```python
from build123d import *

# Parameters (mm, degrees)
BOSS_EXTRUDE1_DEPTH = 304.8
SKETCH3_R           = 2.5
CUT_EXTRUDE2_DEPTH  = 254
SKETCH8_R           = 2.5
CUT_EXTRUDE4_DEPTH  = 254
SKETCH9_R           = 2.25
CUT_EXTRUDE5_DEPTH  = 25.4


with BuildPart() as part:
    # Sketch2 → Boss-Extrude1 (new, symmetric)
    with BuildSketch(Plane.XY):
        with BuildLine():
            Line((-12.7, -12.7), (12.7, -12.7))
            Line((12.7, -12.7), (12.7, 12.7))
            Line((12.7, 12.7), (11.1125, 12.7))
            ThreePointArc((11.1125, 12.7), (9.989967985, 12.235032015), (9.525, 11.1125))
            Line((9.525, 11.1125), (9.525, -6.35))
            ThreePointArc((9.525, -6.35), (8.59506403, -8.59506403), (6.35, -9.525))
            Line((6.35, -9.525), (-11.1125, -9.525))
            ThreePointArc((-11.1125, -9.525), (-12.235032015, -9.989967985), (-12.7, -11.1125))
            Line((-12.7, -11.1125), (-12.7, -12.7))
        make_face()
    extrude(amount=BOSS_EXTRUDE1_DEPTH, both=True)

    # Sketch3 → Cut-Extrude2 (cut)
    with BuildSketch(Plane(origin=(0, 0, 0), x_dir=(1, 0, 0), z_dir=(0, 1, 0))):
        with Locations(Location((-6.35, 285.75, 0), (0, 0, 270))):
            Circle(SKETCH3_R)
        with Locations(Location((0, 292.1, 0), (0, 0, 270))):
            Circle(SKETCH3_R)
        with Locations(Location((0, 266.7, 0), (0, 0, 270))):
            Circle(SKETCH3_R)
        with Locations(Location((0, 228.6, 0), (0, 0, 270))):
            Circle(SKETCH3_R)
        with Locations(Location((0, 190.5, 0), (0, 0, 270))):
            Circle(SKETCH3_R)
        with Locations(Location((0, 152.4, 0), (0, 0, 270))):
            Circle(SKETCH3_R)
        with Locations(Location((0, 114.3, 0), (0, 0, 270))):
            Circle(SKETCH3_R)
        with Locations(Location((0, 76.2, 0), (0, 0, 270))):
            Circle(SKETCH3_R)
        with Locations(Location((0, 38.1, 0), (0, 0, 270))):
            Circle(SKETCH3_R)
        with Locations(Location((0, 0, 0), (0, 0, 270))):
            Circle(SKETCH3_R)
        with Locations(Location((0, -38.1, 0), (0, 0, 270))):
            Circle(SKETCH3_R)
        with Locations(Location((0, -76.2, 0), (0, 0, 270))):
            Circle(SKETCH3_R)
        with Locations(Location((0, -114.3, 0), (0, 0, 270))):
            Circle(SKETCH3_R)
        with Locations(Location((0, -292.1, 0), (0, 0, 270))):
            Circle(SKETCH3_R)
        with Locations(Location((-6.35, -285.75, 0), (0, 0, 270))):
            Circle(SKETCH3_R)
        with Locations(Location((0, -152.4, 0), (0, 0, 270))):
            Circle(SKETCH3_R)
        with Locations(Location((0, -190.5, 0), (0, 0, 270))):
            Circle(SKETCH3_R)
        with Locations(Location((0, -228.6, 0), (0, 0, 270))):
            Circle(SKETCH3_R)
        with Locations(Location((0, -266.7, 0), (0, 0, 270))):
            Circle(SKETCH3_R)
    extrude(amount=-CUT_EXTRUDE2_DEPTH, mode=Mode.SUBTRACT)

    # Sketch8 → Cut-Extrude4 (cut)
    with BuildSketch(Plane(origin=(12.7, 0, -12.7), x_dir=(0, 0, 1), z_dir=(-1, 0, 0))):
        with Locations(Location((295.275, 6.35, 0), (0, 0, 90))):
            Circle(SKETCH8_R)
        with Locations(Location((301.625, 0, 0), (0, 0, 90))):
            Circle(SKETCH8_R)
        with Locations(Location((279.4, 0, 0), (0, 0, 90))):
            Circle(SKETCH8_R)
        with Locations(Location((241.3, 0, 0), (0, 0, 90))):
            Circle(SKETCH8_R)
        with Locations(Location((203.2, 0, 0), (0, 0, 90))):
            Circle(SKETCH8_R)
        with Locations(Location((165.1, 0, 0), (0, 0, 90))):
            Circle(SKETCH8_R)
        with Locations(Location((127, 0, 0), (0, 0, 90))):
            Circle(SKETCH8_R)
        with Locations(Location((88.9, 0, 0), (0, 0, 90))):
            Circle(SKETCH8_R)
        with Locations(Location((50.8, 0, 0), (0, 0, 90))):
            Circle(SKETCH8_R)
        with Locations(Location((12.7, 0, 0), (0, 0, 90))):
            Circle(SKETCH8_R)
        with Locations(Location((-25.4, 0, 0), (0, 0, 90))):
            Circle(SKETCH8_R)
        with Locations(Location((-63.5, 0, 0), (0, 0, 90))):
            Circle(SKETCH8_R)
        with Locations(Location((-101.6, 0, 0), (0, 0, 90))):
            Circle(SKETCH8_R)
        with Locations(Location((-276.225, 0, 0), (0, 0, 90))):
            Circle(SKETCH8_R)
        with Locations(Location((-269.875, 6.35, 0), (0, 0, 90))):
            Circle(SKETCH8_R)
        with Locations(Location((-139.7, 0, 0), (0, 0, 90))):
            Circle(SKETCH8_R)
        with Locations(Location((-177.8, 0, 0), (0, 0, 90))):
            Circle(SKETCH8_R)
        with Locations(Location((-215.9, 0, 0), (0, 0, 90))):
            Circle(SKETCH8_R)
        with Locations(Location((-254, 0, 0), (0, 0, 90))):
            Circle(SKETCH8_R)
    extrude(amount=CUT_EXTRUDE4_DEPTH, mode=Mode.SUBTRACT)

    # Sketch9 → Cut-Extrude5 (cut)
    with BuildSketch(Plane(origin=(0, -12.7, 0), x_dir=(0, 0, -1), z_dir=(0, 1, 0))):
        with Locations(Location((-16, 0, 0), (0, 0, 270))):
            Circle(SKETCH9_R)
        with Locations(Location((16, 0, 0), (0, 0, 270))):
            Circle(SKETCH9_R)
    extrude(amount=CUT_EXTRUDE5_DEPTH, mode=Mode.SUBTRACT)


solid = part.part
```
CAD build for the part. Positions are in the model's coordinates, mm. A direction names the side the tool comes from. Coordinates: 2 decimals unless noted, no trailing zeros. Use a Markdown table: item, result. Add a question column.
(1) Drill centre lines: line 1 along X through (y, z) = (-11.2, 16); line 2 along Y through (x, z) = (4, -186.5) (3 decimals); line 3 along X through (y, z) = (4, -199) (3 decimals). Where is each one in solid material? Low to high. Write a range as [from, to].
(2) Which spindle directions (+Z, -Z, +X, -X, +Y, -Y) get a long thin tool onto all of the face, cutting with end or side? Do faces 1 (the face through (-2, -9.525, 4)), 2 (the face through (0, -12.7, 4)). Say none if no direction does.
(3) Flat gauge pins, fed straight in: pin 1 (6.5 mm diameter, centred on y = 6.35, z = 282.575, fed in from +X); pin 2 (2 mm diameter, centred on x = 3.5, z = -150.5, fed in from +Y) (3 decimals); pin 3 (3 mm diameter, centred on y = 0, z = -76.2, fed in from +X); pin 4 (8 mm diameter, centred on y = 0, z = 0, fed in from -X) (3 decimals). Where does each tip first touch, or does it go through?
Solved:
| question | item | result |
|---|---|---|
| 1 | line 1 | x = [-12.7, -2.25], [2.25, 12.7] |
| 1 | line 2 | y = [-12.7, -9.525] |
| 1 | line 3 | x = [9.525, 12.7] |
| 2 | face 1 | +Z, -Z, -X, +Y |
| 2 | face 2 | +Z, -Z, +X, -X, -Y |
| 3 | pin 1 | stops at x = 12.7 |
| 3 | pin 2 | stops at y = -9.525 |
| 3 | pin 3 | passes through |
| 3 | pin 4 | stops at x = 9.525 |
